Work out the finished part from the listing and answer in its coordinate system (mm). Round coordinates to 2 decimals unless told otherwise and drop trailing zeros. Order: outer loops, then holes, each group sorted by start corner. A loop starts at its lowest first (then second) coordinate and runs counter-clockwise, first axis right, second up. Notation, with made-up numbers: (50.25, 53.5) - (65.25, 53.5) arc R27 cw to (65.25, 70.5) - close; hole circle Ø8 at (84, -23). An arc over 180 degrees is marked (long way). Use CSV: the item, a comma, the result in double quotes.
from build123d import *

# Parameters (mm, degrees)
CROQUIS1_W              = 30
CROQUIS1_H              = 28
CROQUIS1_W_2            = 10
CROQUIS1_H_2            = 25
SALIENTE_EXTRUIR2_DEPTH = 3


with BuildPart() as part:
    # Croquis1 → Saliente-Extruir2 (new body)
    with BuildSketch(Plane(origin=(0, 0, 0), x_dir=(1, 0, 0), z_dir=(0, 1, 0))):
        Polygon((0, 0), (15, 0), (15, 3), (35, 3), (35, 0), (265, 0), (265, 3), (285, 3), (285, 0), (300, 0), (300, 15), (297, 15), (297, 35), (300, 35), (300, 265), (297, 265), (297, 285), (300, 285), (300, 300), (285, 300), (285, 297), (265, 297), (265, 300), (35, 300), (35, 297), (15, 297), (15, 300), (0, 300), (0, 285), (3, 285), (3, 265), (0, 265), (0, 35), (3, 35), (3, 15), (0, 15), align=None)
        with Locations((150, 150)):
            Rectangle(CROQUIS1_W, CROQUIS1_H, mode=Mode.SUBTRACT)
        with Locations((176.5, 150)):
            Rectangle(CROQUIS1_W_2, CROQUIS1_H_2, mode=Mode.SUBTRACT)
    extrude(amount=SALIENTE_EXTRUIR2_DEPTH)


solid = part.part
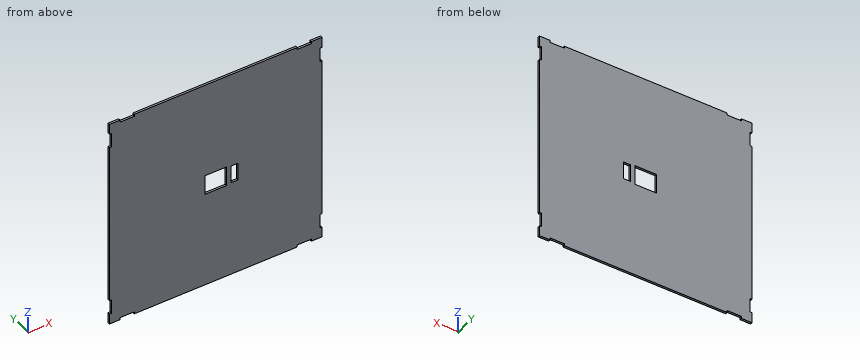
(1) Find section C-C (z = -274). Determine the outline of the cut face in (x, y).
Findings below:
outline,"(3, 0) - (297, 0) - (297, 3) - (3, 3) - close"
(2) Each of these flat-tipped pins is pushed along its axis until it touches: pin 1 (0.9 mm diameter, centred on x = 2, y = 1, fed in from +Z); pin 2 (0.9 mm diameter, centred on y = 2, z = -27, fed in from -X); pin 3 (1.5 mm diameter, centred on x = 273.5, y = 1.5, fed in from -Z). Where does it stop, or does it pass through?
Findings below:
pin 1,"stops at z = 0"
pin 2,"stops at x = 3"
pin 3,"stops at z = -297"
(3) Find section A-A (x = 153.5). Determine the outline of the cut face in (y, z), and give its area (3 significant figures).
Findings below:
outline,"(0, -300) - (3, -300) - (3, -164) - (0, -164) - close; (0, -136) - (3, -136) - (3, 0) - (0, 0) - close"
area,"816 mm²"
(4) Find the intervals of material crossed by L1, parallel to X at y = 0.2, z = -142; L2, parallel to Z at x = 155, y = 1.6; L3, parallel to X at y = 2.2, z = -271.5, in increasing order. Write a range as from..to.
Findings below:
L1,"x = 0..135, 165..171.5, 181.5..300"
L2,"z = -300..-164, -136..0"
L3,"x = 3..297"
(5) Find section B-B (y = 1.15). State how many separate pieces and enclosed holes the cut face has, and give its area (3 significant figures).
Findings below:
separate pieces,"1"
enclosed holes,"2"
area,"88,400 mm²"
